Design review of the part built by this model. Coordinates are the model's own, in mm. A direction names the side the tool comes from. Give positions to 0.01 mm unless a question says otherwise; leave off trailing zeros. Loops run counter-clockwise (first coordinate to the right, second up) from the corner with the lowest first, then second, coordinate; pieces in that order, holes last. Notation, with made-up numbers: M 3,-12 L 7,-12 A17 ccw 7,11 Z; hole C 10,41.25 d7. An arc over 180 degrees is marked long. Use one line per item in the form item = value. Start each with the question number.
from build123d import *

# Parameters (mm, degrees)
CYLINDER_R     = 2.75
CYLINDER_DEPTH = 10
SKETCH_R       = 1.7
PAD_DEPTH      = 5
FILLET_R       = 1


with BuildPart() as cylinder:
    # Cylinder → Cylinder (new body)
    with BuildSketch(Plane.XY.offset(2.5)):
        Circle(CYLINDER_R)
    extrude(amount=CYLINDER_DEPTH)


with BuildPart() as fillet_body:
    # Sketch → Pad (new body)
    with BuildSketch(Plane.XY):
        with BuildLine():
            ThreePointArc((0.526316, -4.972222), (5, 0), (0.526316, 4.972222))
            Line((-8.868441, 5.966669), (0.526316, 4.972222))
            ThreePointArc((-8.868441, 5.966669), (-15.5, -1e-05), (-8.868421, -5.966666))
            Line((0.526316, -4.972222), (-8.868421, -5.966666))
        make_face()
        Circle(SKETCH_R, mode=Mode.SUBTRACT)
    extrude(amount=PAD_DEPTH)

    # Cut: cut Cylinder
    add(cylinder.part, mode=Mode.SUBTRACT)

    # Fillet
    fillet_edges = [fillet_body.edges().sort_by_distance(p)[0] for p in [
        (5, 0, 5),
        (-4.171053, -5.469444, 5),
        (-4.171063, 5.469445, 5),
        (-15.5, -1e-05, 5),
        (-2.75, 0, 5),
    ]]
    fillet(fillet_edges, radius=FILLET_R)


solid = fillet_body.part
Q1. Take a section at B-B on z = 3.5. Give the boundary of the cut face in (x, y), plus the area to 3 significant figures.
Q2. For faces 4 (the flat face through (-9, 0, 5)), 5 (the cylindrical face through (-0.596, -2.685, 3.24)), list the 3-axis set-ups (+Z, -Z, +X, -X, +Y, -Y) from which the entire face can be reached by the end or side of a thin tool; tool diameter is ignored.
Q3. Take a section at A-A on z = 1.75. Give the boundary of the cut face in (x, y), plus the area to 3 significant figures.
Q4. Wall thickness on probe 1 along Y at (x, z) = (0, 1.85); probe 2 along Y at (x, z) = (0, 2.9); probe 3 along Z at (x, y) = (0.75, -1.75): over which ranges is each line inside the solid? List them lowest first.
Q5. Clearance check with flat-ended pins moving along their axes: pin 1 Ø6 at (x, y) = (-0.5, 0) entering from +Z; pin 2 Ø1 at (y, z) = (-2, 1) entering from +X. State where each tip first meets the part, or that it passes through.
Q6. The part is to be moulded in two halves that separate along Y. For faces 1 (the cylindrical face through (-4.14, -5.18, 4.7)), 2 (the flat face through (-5, 0, 0)), 3 (the cylindrical face through (-0.37, -1.66, 1.23)), say which applies: pulls with the +Y half, pulls with the -Y half, needs draft (parallel to the pull), parting line crosses it, or undercut.
Response values:
q1.outline = M -8.87,-5.97 L 0.53,-4.97 A5 ccw 0.53,4.97 L -8.87,5.97 A6 ccw long Z; hole C 0,0 d5.5
q1.area = 177 mm^2
q2.face_4 = +Z, +X, -X, +Y, -Y
q2.face_5 = +Z
q3.outline = M -8.87,-5.97 L 0.53,-4.97 A5 ccw 0.53,4.97 L -8.87,5.97 A6 ccw long Z; hole C 0,0 d3.4
q3.area = 192 mm^2
q4.probe_1 = -5.03 to -1.7, 1.7 to 5.03
q4.probe_2 = -5.03 to -2.75, 2.75 to 5.03
q4.probe_3 = 0 to 2.5
q5.pin_1 = 4.97
q5.pin_2 = 4.77
q6.face_1 = pulls with the -Y half
q6.face_2 = needs draft
q6.face_3 = undercut
